Here's how the part is built. I have some questions about the finished solid (model axes, mm). A direction names the side the tool comes from. Coordinates: 2 decimals unless noted, no trailing zeros. Write each loop counter-clockwise with the first axis right and the second up, starting at its lowest first coordinate (ties: lowest second). Pieces come first, ordered by that corner, then holes.
Item 1: If I drill on line 1 (X direction, y = 0.1, z = -20.75); line 2 (Z direction, x = -2.3, y = 1); line 3 (X direction, y = -0.9, z = -12.5), over which ranges is the centre line in solid material (lowest first)?
Item 2: I'm going to push flat-ended pins straight in: pin 1 Ø1 at (x, y) = (0.5, 0) entering from +Z; pin 2 Ø2 at (x, z) = (2, -3.5) entering from -Y; pin 3 Ø2 at (x, y) = (1, 1.5) entering from -Z. Where does each tip first touch, or does it pass through?
Item 3: If we section it at B-B (z = -4.5): Please give me the cut outline in (x, y) (3 decimals).
Item 4: We'd pull the mould along Y, two halves only. Please class faces 4 (the face through (-2.685, -0.596, 1.482)), 5 (the face through (-1, 2, 0)), 6 (the face through (0.63, 1.08, 2.16)): +Y half, -Y half, draft (parallel to the pull), parting line (faces both ways), or undercut.
Item 5: For faces 1 (the face through (0, 0, -22)), 2 (the face through (-0.618, 1.087, 2.16)), 3 (the face through (-1.43, -0.32, -11.15)), which set-ups out of +Z, -Z, +X, -X, +Y, -Y let a thin tool reach every point of the face, with its end or its side?
Item 6: If we section it at A-A (y = 0): Please give me the cut outline in (x, z) (3 decimals), then the cut area to 3 significant figures.
from build123d import *

# Parameters (mm, degrees)
SCHNITT_LINEAR_AUSTRAGEN1_DEPTH = 1.8
FASE1_SIZE                      = 0.2
VERRUNDUNG1_R                   = 0.2
VERRUNDUNG2_R                   = 0.1


with BuildPart() as part:
    # Skizze1 → Rotation1 (revolve)
    with BuildSketch(Plane(origin=(0, 0, 0), x_dir=(0, 0, -1), z_dir=(1, 0, 0))):
        Polygon((-3, 0), (-3, 2.75), (0, 2.75), (0, 1.465), (22, 1.465), (22, 0), align=None)
    revolve(axis=Axis((0, 0, 21.919879518), (0, 0, -1)))

    # Skizze2 → Schnitt-Linear austragen1 (cut)
    with BuildSketch(Plane.XY.offset(3)):
        Polygon((1.25, -0.721687836), (1.25, 0.721687836), (0, 1.443375673), (-1.25, 0.721687836), (-1.25, -0.721687836), (0, -1.443375673), align=None)
    extrude(amount=-SCHNITT_LINEAR_AUSTRAGEN1_DEPTH, mode=Mode.SUBTRACT)

    # Fase1
    fase1_edges = [part.edges().sort_by_distance(p)[0] for p in [
        (0, -1.465, -22),
        (0, -2.75, 0),
        (0, -2.75, 3),
    ]]
    chamfer(fase1_edges, length=FASE1_SIZE)

    # Verrundung1
    verrundung1_edges = [part.edges().sort_by_distance(p)[0] for p in [
        (0.625, -1.082531755, 1.2),
        (1.25, -0.721687836, 2.1),
        (-0.625, -1.082531755, 1.2),
        (0, -1.443375673, 2.1),
        (-1.25, 0, 1.2),
        (-1.25, -0.721687836, 2.1),
        (-0.625, 1.082531755, 1.2),
        (-1.25, 0.721687836, 2.1),
        (0.625, 1.082531755, 1.2),
        (0, 1.443375673, 2.1),
        (1.25, 0, 1.2),
        (1.25, 0.721687836, 2.1),
        (0, -1.465, 0),
    ]]
    fillet(verrundung1_edges, radius=VERRUNDUNG1_R)

    # Verrundung2
    verrundung2_edges = [part.edges().sort_by_distance(p)[0] for p in [
        (-0.625, -1.082531755, 3),
        (-1.25, 0, 3),
        (-0.625, 1.082531755, 3),
        (0.625, 1.082531755, 3),
        (1.25, 0, 3),
        (0.625, -1.082531755, 3),
        (-1.223205081, -0.706217783, 3),
        (0, -1.412435565, 3),
        (1.223205081, -0.706217783, 3),
        (1.223205081, 0.706217783, 3),
        (0, 1.412435565, 3),
        (-1.223205081, 0.706217783, 3),
    ]]
    fillet(verrundung2_edges, radius=VERRUNDUNG2_R)


solid = part.part
Answer list:
1. line 1: x = -1.46 to 1.46
1. line 2: z = 0 to 3
1. line 3: x = -1.16 to 1.16
2. pin 1: stops at z = 1.2
2. pin 2: stops at y = -1.07
2. pin 3: stops at z = -22
3. outline: circle Ø2.93 at (0, 0)
4. face 4: parting line
4. face 5: draft
4. face 6: undercut
5. face 1: -Z, +X, -X, +Y, -Y
5. face 2: +Z
5. face 3: -Z
6. outline: (-2.75, 0.2) - (-2.55, 0) - (-1.665, 0) arc R0.2 cw to (-1.465, -0.2) - (-1.465, -21.8) - (-1.265, -22) - (1.265, -22) - (1.465, -21.8) - (1.465, -0.2) arc R0.2 cw to (1.665, 0) - (2.55, 0) - (2.75, 0.2) - (2.75, 2.8) - (2.55, 3) - (1.35, 3) arc R0.1 ccw to (1.25, 2.9) - (1.25, 1.4) arc R0.2 cw to (1.05, 1.2) - (-1.05, 1.2) arc R0.2 cw to (-1.25, 1.4) - (-1.25, 2.9) arc R0.1 ccw to (-1.35, 3) - (-2.55, 3) - (-2.75, 2.8) - close
6. area: 76.4 mm2
